Geometry: final body of the model. Coordinates: model frame, mm. A direction names the side the tool comes from. Round coordinates to 2 decimals unless told otherwise and drop trailing zeros. Loops run counter-clockwise (first coordinate to the right, second up) from the corner with the lowest first, then second, coordinate; pieces in that order, holes last. Notation, with made-up numbers: (-24.75, -3.5) - (6.25, -3.5) arc R9 ccw to (6.25, 13.5) - close; hole circle Ø6 at (12.25, 29). An arc over 180 degrees is marked (long way). Return JSON: item names as keys, results as strings. Group by question number.
1. Draft query along X for faces 1 (the face through (68, -1, 48.26)), 2 (the face through (-2, 1, 0)). Return one class per face: +X half, -X half, draft (parallel to the pull), parting line (faces both ways), or undercut.
2. First-contact query: pin 1 Ø10 at (x, y) = (-72.5, 36) entering from -Z; pin 2 Ø14.5 at (x, y) = (-75.5, -47) entering from +Z. Flat tips, straight axial feed; report the tip coordinate or a pass-through.
3. Section B-B on x = -5. Return loops of the section in (y, z), and give its area (3 significant figures).
4. Set-up query: faces 3 (the face through (-2, -88.9, 25)), 4 (the face through (68, 55, 48.26)), 5 (the face through (82, -21.418, 3)). Return all of +Z, -Z, +X, -X, +Y, -Y with unobstructed straight access to the full face (end or side cutting, diameter ignored); none if empty.
5. Section C-C on x = 74. Return loops of the section in (y, z), and give its area (3 significant figures).
6. Section A-A on y = 42.5. Return loops of the section in (x, z).
7. Material intervals for probe 1 along Z at (x, y) = (-52, -63); probe 2 along Z at (x, y) = (-16, -68), sorted ascending.
from build123d import *

# Parameters (mm, degrees)
SKETCH1_W           = 215.9
SKETCH1_H           = 177.8
BOSS_EXTRUDE1_DEPTH = 50.8
SKETCH2_W           = 47.801549888
SKETCH2_H           = 50.8
CUT_EXTRUDE1_DEPTH  = 2.54
SKETCH3_W           = 50.8
SKETCH3_H           = 50.8
CUT_EXTRUDE2_DEPTH  = 5.08


with BuildPart() as part:
    # Sketch1 → Boss-Extrude1 (new body)
    with BuildSketch(Plane.XY):
        Rectangle(SKETCH1_W, SKETCH1_H)
    extrude(amount=BOSS_EXTRUDE1_DEPTH)

    # Sketch2 → Cut-Extrude1 (cut)
    with BuildSketch(Plane.XY.offset(50.8)):
        with Locations((-0.538457271, 55.022877852)):
            Rectangle(SKETCH2_W, SKETCH2_H)
        with Locations((-69.118457271, 55.022877852)):
            Rectangle(SKETCH2_W, SKETCH2_H)
        with Locations((68.041542729, 55.022877852)):
            Rectangle(SKETCH2_W, SKETCH2_H)
        with Locations((-69.118457271, -0.857122148)):
            Rectangle(SKETCH2_W, SKETCH2_H)
        with Locations((-0.538457271, -0.857122148)):
            Rectangle(SKETCH2_W, SKETCH2_H)
        with Locations((68.041542729, -0.857122148)):
            Rectangle(SKETCH2_W, SKETCH2_H)
        with Locations((-69.118457271, -56.737122148)):
            Rectangle(SKETCH2_W, SKETCH2_H)
        with Locations((-0.538457271, -56.737122148)):
            Rectangle(SKETCH2_W, SKETCH2_H)
        with Locations((68.041542729, -56.737122148)):
            Rectangle(SKETCH2_W, SKETCH2_H)
    extrude(amount=-CUT_EXTRUDE1_DEPTH, mode=Mode.SUBTRACT)

    # Sketch3 → Cut-Extrude2 (cut)
    with BuildSketch(Plane(origin=(0, 0, 0), x_dir=(-1, 0, 0), z_dir=(0, 0, -1))):
        with Locations((58.475064597, 54.782080131)):
            Rectangle(SKETCH3_W, SKETCH3_H)
        with Locations((58.475064597, -59.517919869)):
            Rectangle(SKETCH3_W, SKETCH3_H)
        with Locations((-81.224935403, 3.982080131)):
            Rectangle(SKETCH3_W, SKETCH3_H)
    extrude(amount=-CUT_EXTRUDE2_DEPTH, mode=Mode.SUBTRACT)


solid = part.part
Taken from the geometry:
{
 "1": {"face 1": "undercut", "face 2": "draft"},
 "2": {"pin 1": "z = 5.08", "pin 2": "z = 48.26"},
 "3": {"outline": "(-88.9, 0) - (88.9, 0) - (88.9, 50.8) - (80.42, 50.8) - (80.42, 48.26) - (29.62, 48.26) - (29.62, 50.8) - (24.54, 50.8) - (24.54, 48.26) - (-26.26, 48.26) - (-26.26, 50.8) - (-31.34, 50.8) - (-31.34, 48.26) - (-82.14, 48.26) - (-82.14, 50.8) - (-88.9, 50.8) - close", "area": "8,650 mm2"},
 "4": {"face 3": "+Z, -Z, +X, -X, -Y", "face 4": "+Z", "face 5": "-Z"},
 "5": {"outline": "(-88.9, 0) - (-21.42, 0) - (-21.42, 5.08) - (29.38, 5.08) - (29.38, 0) - (88.9, 0) - (88.9, 50.8) - (80.42, 50.8) - (80.42, 48.26) - (29.62, 48.26) - (29.62, 50.8) - (24.54, 50.8) - (24.54, 48.26) - (-26.26, 48.26) - (-26.26, 50.8) - (-31.34, 50.8) - (-31.34, 48.26) - (-82.14, 48.26) - (-82.14, 50.8) - (-88.9, 50.8) - close", "area": "8,390 mm2"},
 "6": {"outline": "(-107.95, 0) - (-83.88, 0) - (-83.88, 5.08) - (-33.08, 5.08) - (-33.08, 0) - (107.95, 0) - (107.95, 50.8) - (91.94, 50.8) - (91.94, 48.26) - (44.14, 48.26) - (44.14, 50.8) - (23.36, 50.8) - (23.36, 48.26) - (-24.44, 48.26) - (-24.44, 50.8) - (-45.22, 50.8) - (-45.22, 48.26) - (-93.02, 48.26) - (-93.02, 50.8) - (-107.95, 50.8) - close"},
 "7": {"probe 1": "5.08 to 48.26", "probe 2": "0 to 48.26"}
}
